CAD build for the part. Positions are in the model's coordinates, mm. Coordinates: 2 decimals unless noted, no trailing zeros. Loops run counter-clockwise (first coordinate to the right, second up) from the corner with the lowest first, then second, coordinate; pieces in that order, holes last. Notation, with made-up numbers: (44.5, 18) -> (71.5, 18) arc R17 cw to (71.5, 41) -> close; hole circle Ø4 at (48.5, 73). An arc over 180 degrees is marked (long way). Write each question's results on one line, items separated by ' | '.
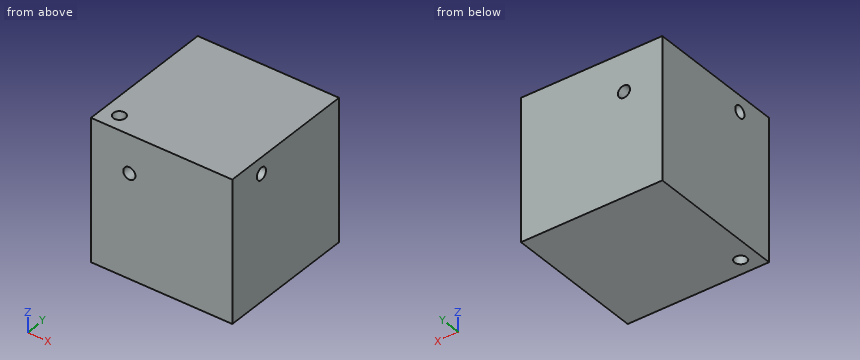
Autodesk Inventor part; units mm, degrees
ref_plane "YZ Plane" through (0, 0, 0) normal (1, 0, 0) x (0, 1, 0)
ref_plane "XZ Plane" through (0, 0, 0) normal (0, 1, 0) x (-1, 0, 0)
ref_plane "XY Plane" through (0, 0, 0) normal (0, 0, 1) x (1, 0, 0)
sketch "Sketch1" plane through (0, 0, 0) normal (0, 0, 1) x (1, 0, 0)
  line L0 (0, 0) -> (0, 70)
  line L1 (0, 70) -> (70, 70)
  line L2 (70, 70) -> (70, 0)
  line L3 (70, 0) -> (0, 0)
  dimension "d0" = 70
  dimension "d1" = 70
extrude "Extrusion1" add sketch "Sketch1" along normal blind 70
sketch "Sketch2" plane through (0, 0, 70) normal (0, 0, 1) x (1, 0, 0)
  circle A0 centre (8, 8) radius 3
  dimension "d6" = 6
hole "Hole1" at (8, 8, 70) direction (0, 0, -1) diameter 6 end through all
sketch "Sketch3" plane through (0, 0, 0) normal (-1, 0, 0) x (0, 0, 1)
  line L0 (69.699, 0) -> (70, 18.9976)
  line L1 (70, 70) -> (70, 0)
  line L2 (70, 18.9976) -> (62.001, 19.1244)
  circle A0 centre (62.001, 19.1244) radius 3
  point P0 (0, 0)
  dimension "d14" = 19
  dimension "d15" = 8
  dimension "d16" = 6
hole "Hole2" at (0, 19.1244, 62.001) direction (1, 0, 0) diameter 6 end through all
sketch "Sketch4" plane through (0, 70, 0) normal (0, 1, 0) x (1, 0, 0)
  line L0 (0, -70.1804) -> (0, -51.1804)
  line L1 (0, 0) -> (0, -70)
  line L2 (0, -51.1804) -> (19, -51.1804)
  circle A0 centre (19, -51.1804) radius 3
  dimension "d24" = 19
  dimension "d25" = 19
  dimension "d26" = 6
hole "Hole3" at (19, 70, 51.1804) direction (0, -1, 0) diameter 6 end through all
properties part number "Bundhjørne1" material "PC/ABS Plastic"
1) Slice it at B-B (x = 8). Write the cut outline in (y, z).
Outcome:
outline: (0, 0) -> (5, 0) -> (5, 70) -> (0, 70) -> close; (11, 0) -> (70, 0) -> (70, 70) -> (11, 70) -> close; hole circle Ø6 at (19.12, 62)
2) Slice it at A-A (y = 8). Write the cut outline in (x, z), then the cut area to 3 significant figures.
Outcome:
outline: (0, 0) -> (5, 0) -> (5, 70) -> (0, 70) -> close; (11, 0) -> (70, 0) -> (70, 70) -> (11, 70) -> close; hole circle Ø6 at (19, 51.18) | area: 4,450 mm^2
3) Drill centre lines: L1, parallel to Z at x = 19, y = 19; L2, parallel to X at y = 8, z = 56. Where is each one in solid material? Low to high. Write a range as from..to.
Outcome:
L1: z = 0..48.18, 54.18..59, 65..70 | L2: x = 0..5, 11..70
